Input: part model. Units: mm. Frame: model coordinates. A direction names the side the tool comes from. Give positions to 0.01 mm unless a question says otherwise; leave off trailing zeros. Loops run counter-clockwise (first coordinate to the right, second up) from the corner with the lowest first, then second, coordinate; pieces in that order, holes last. Notation, with made-up numbers: (43.25, 68.25) - (91.25, 68.25) arc R7 cw to (91.25, 77.25) - close; hole circle Ø11 at (-15.75, 47). An arc over 180 degrees is marked (long way). Answer as a JSON object with one key per item and string values.
from build123d import *

# Parameters (mm, degrees)
BOSS_EXTRUDE1_DEPTH = 2.975
SKETCH3_R           = 2.175
CUT_EXTRUDE1_DEPTH  = 10
BOSS_EXTRUDE2_DEPTH = 3
CUT_EXTRUDE4_DEPTH  = 3
CUT_EXTRUDE5_DEPTH  = 3
CUT_EXTRUDE6_DEPTH  = 3
CUT_EXTRUDE7_DEPTH  = 3


with BuildPart() as part:
    # Sketch1 → Boss-Extrude1 (new body)
    with BuildSketch(Plane(origin=(0, 0, 0), x_dir=(1, 0, 0), z_dir=(0, 1, 0))):
        with BuildLine():
            Line((-23.171929825, 5.625877193), (-23.171929825, -7.074122807))
            Line((-23.171929825, -7.074122807), (2.228070175, -7.074122807))
            ThreePointArc((2.228070175, -7.074122807), (8.578070175, -0.724122807), (2.228070175, 5.625877193))
            Line((2.228070175, 5.625877193), (-23.171929825, 5.625877193))
        make_face()
    extrude(amount=BOSS_EXTRUDE1_DEPTH)

    # Sketch3 → Cut-Extrude1 (cut)
    with BuildSketch(Plane(origin=(0, 2.975, 0), x_dir=(1, 0, 0), z_dir=(0, 1, 0))):
        Polygon((-17.882133224, 5.625877193), (-21.171929825, 5.625877193), (-20.476894991, 4.187255521), (-18.476894991, 4.187255521), align=None)
        Polygon((-12.382133224, 5.625877193), (-15.671929825, 5.625877193), (-14.976894991, 4.187255521), (-12.976894991, 4.187255521), align=None)
        Polygon((-6.882133224, 5.625877193), (-10.171929825, 5.625877193), (-9.476894991, 4.187255521), (-7.476894991, 4.187255521), align=None)
        Polygon((-1.382133224, 5.625877193), (-4.671929825, 5.625877193), (-3.976894991, 4.187255521), (-1.976894991, 4.187255521), align=None)
        with Locations(Location((-9.806894991, -0.713854538, 0), (0, 0, 270))):
            Circle(SKETCH3_R)
    extrude(amount=-CUT_EXTRUDE1_DEPTH, mode=Mode.SUBTRACT)

    # Sketch4 → Boss-Extrude2 (add)
    with BuildSketch(Plane(origin=(0, 2.975, 0), x_dir=(1, 0, 0), z_dir=(0, 1, 0))):
        Polygon((2.012508497, 5.625877193), (2.877447204, 5.848143738), (4.955403332, 6.631142622), (6.932313313, 7.831153974), (7.181023471, 7.907898717), (7.449388225, 7.917059752), (7.669017249, 7.869526346), (7.909998428, 7.749936115), (8.090301913, 7.593296768), (8.229089145, 7.396943716), (8.320584378, 7.15885929), (8.349013293, 6.921336926), (7.506024116, 3.278478183), (7.381859278, 2.936726049), (7.191829205, 3.236129243), (6.188322225, 4.239636223), (4.955403332, 5.010347862), (3.635222185, 5.468003098), align=None)
    extrude(amount=-BOSS_EXTRUDE2_DEPTH)

    # Sketch5 → Cut-Extrude4 (cut)
    with BuildSketch(Plane.XZ):
        Polygon((7.381859278, -2.936726049), (6.307567975, 0.076195893), (5.651690171, 1.50143626), (4.463765556, 3.356436211), (2.862913669, 4.934447261), (1.01921029, 6.082107474), (-1.092761509, 6.819455434), (-3.321732513, 7.068870042), (2.228070175, 7.074122807), (3.760260473, 6.886500018), (5.204465919, 6.333362361), (6.48158413, 5.439005525), (7.484091138, 4.287371835), (8.1884819, 2.914098165), (8.543501486, 1.385808052), (8.521355854, -0.122668414), (8.123713387, -1.634667375), (7.393611108, -2.969071864), align=None)
    extrude(amount=-CUT_EXTRUDE4_DEPTH, mode=Mode.SUBTRACT)

    # Sketch8 → Cut-Extrude5 (cut)
    with BuildSketch(Plane.XZ):
        Polygon((7.393611108, -2.969071864), (4.817266947, 7.178326075), (13.149056149, 1.259568719), align=None)
    extrude(amount=-CUT_EXTRUDE5_DEPTH, mode=Mode.SUBTRACT)

    # Sketch9 → Cut-Extrude6 (cut)
    with BuildSketch(Plane(origin=(0, 2.975, 0), x_dir=(1, 0, 0), z_dir=(0, 1, 0))):
        Polygon((-2.812690859, -7.210619116), (5.027177804, -8.631982179), (5.504181298, -6.000955074), align=None)
    extrude(amount=-CUT_EXTRUDE6_DEPTH, mode=Mode.SUBTRACT)

    # Sketch10 → Cut-Extrude7 (cut)
    with BuildSketch(Plane(origin=(0, 2.975, 0), x_dir=(1, 0, 0), z_dir=(0, 1, 0))):
        Polygon((-3.321732513, -7.068870042), (-3.353757598, -7.074122807), (-1.90048619, -7.144223144), (-1.755238834, -7.012343357), align=None)
    extrude(amount=-CUT_EXTRUDE7_DEPTH, mode=Mode.SUBTRACT)


solid = part.part
Item 1: Cut plane D-D (x = 1.5). Return loops of the section in (y, z) (3 decimals), then the cut area to 3 significant figures.
Geometry check:
{"outline": "(0, -5.626) - (2.975, -5.626) - (2.975, 5.783) - (0, 5.783) - close", "area": "33.9 mm2"}
Item 2: Contact query for flat-ended pins moving along their axis: P1, Ø4, axis at x = -5.5, z = 3, coming from the -Y side; P2, Ø1.1, axis at x = -11, y = 2, coming from the -Z side; P3, Ø1.6, axis at x = -8.5, y = 1, coming from the -Z side. Output: stop coordinate, or through.
Geometry check:
{"P1": "stops at y = 0", "P2": "stops at z = -5.63", "P3": "stops at z = -4.19"}
Item 3: Material intervals for line 1 (X direction, y = 1.5, z = -4.25); line 2 (Y direction, x = 2, z = -1) (3 decimals); line 3 (X direction, y = 1.05, z = -5.25), sorted ascending. Write a range as [from, to].
Geometry check:
{"line 1": "x = [-23.17, -20.51], [-18.45, -15.01], [-12.95, -9.51], [-7.45, -4.01], [-1.95, 7.73]", "line 2": "y = [0, 2.975]", "line 3": "x = [-23.17, -20.99], [-18.04, -15.49], [-12.54, -9.99], [-7.04, -4.49], [-1.54, 7.96]"}
Item 4: Mould query, pull axis Z, two halves, no side actions, for faces 4 (the face through (5.984, 1.467, 0.779)), 5 (the face through (-11.736, 1.508, 1.717)), 6 (the face through (-7, 2.975, -1)). Classes: released by +Z, released by -Z, zero draft, split by the parting line, or undercut.
Geometry check:
{"face 4": "released by +Z", "face 5": "undercut", "face 6": "zero draft"}
Item 5: Cut plane C-C (z = -1.75). Return loops of the section in (x, y) (3 decimals), then the cut area to 3 significant figures.
Geometry check:
{"outline": "(-23.172, 0) - (6.959, 0) - (6.959, 2.975) - (-23.172, 2.975) - close", "area": "89.6 mm2"}
Item 6: Access query for faces 1 (the face through (-9.83, 1.51, -4.92)), 2 (the face through (-11, 1, -5.626)), 3 (the face through (-23.172, 1, 1)). Directions: +Z, -Z, +X, -X, +Y, -Y. A direction counts if a zero-diameter tool reaches every point of the face in a straight line with its end or side. Return the directions, or none.
Geometry check:
{"face 1": "-Z, +Y, -Y", "face 2": "-Z, -X, +Y, -Y", "face 3": "+Z, -Z, -X, +Y, -Y"}
Item 7: Cut plane A-A (x = -11). Return loops of the section in (y, z) (3 decimals), then the cut area to 3 significant figures.
Geometry check:
{"outline": "(0, -5.626) - (2.975, -5.626) - (2.975, -1.105) - (0, -1.105) - close; (0, 2.532) - (2.975, 2.532) - (2.975, 7.074) - (0, 7.074) - close", "area": "27.0 mm2"}
Item 8: Cut plane B-B (z = 0.5). Return loops of the section in (x, y) (3 decimals).
Geometry check:
{"outline": "(-23.172, 0) - (-11.971, 0) - (-11.971, 2.975) - (-23.172, 2.975) - close; (-7.642, 0) - (6.113, 0) - (6.113, 2.975) - (-7.642, 2.975) - close"}
